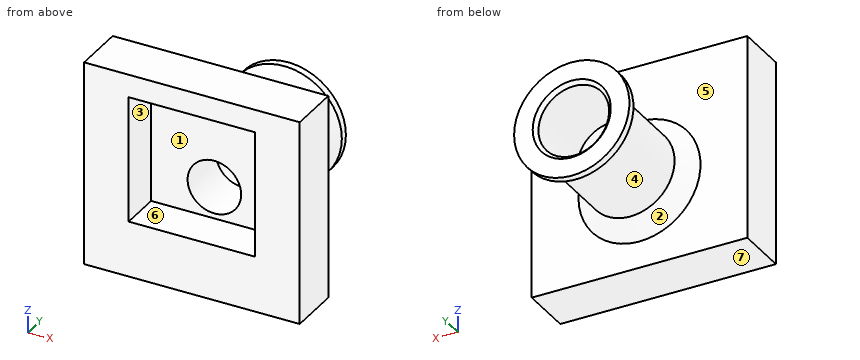
```python
from build123d import *

# Parameters (mm, degrees)
SKETCH2_OUTSIDE_W       = 59.31
SKETCH2_OUTSIDE_H       = 59.31
SKETCH2_OUTSIDE_W_2     = 28.986815524
SKETCH2_OUTSIDE_H_2     = 27.563826398
CUT_EXTRUDE1_DEPTH      = 11
CUT_EXTRUDE1_DEPTH_BACK = 14.593473012
SKETCH3_W               = 17
SKETCH3_H               = 17
CUT_EXTRUDE2_DEPTH      = 6.5


with BuildPart() as part:
    # Sketch1 → Revolve1 (revolve)
    with BuildSketch(Plane.XY):
        Polygon((4.75, 9.5), (4.75, 0), (3.6, -1.15), (3.6, -13.593473012), (22, -13.593473012), (22, -6.593473012), (8.200842899, -6.593473012), (5.95, -4.342630114), (5.95, 7.2), (7.75, 9), (7.75, 10), (5.25, 10), align=None)
    revolve(axis=Axis((0, -12.923275862, 0), (0, 1, 0)))

    # Sketch2 outside → Cut-Extrude1 (cut, two sides)
    with BuildSketch(Plane(origin=(0, 0, 0), x_dir=(1, 0, 0), z_dir=(0, 1, 0))) as cut_extrude1_sk:
        Rectangle(SKETCH2_OUTSIDE_W, SKETCH2_OUTSIDE_H)
        with Locations((0, -2)):
            Rectangle(SKETCH2_OUTSIDE_W_2, SKETCH2_OUTSIDE_H_2, mode=Mode.SUBTRACT)
    extrude(amount=CUT_EXTRUDE1_DEPTH, mode=Mode.SUBTRACT)
    extrude(cut_extrude1_sk.sketch, amount=-CUT_EXTRUDE1_DEPTH_BACK, mode=Mode.SUBTRACT)

    # Sketch3 → Cut-Extrude2 (cut)
    with BuildSketch(Plane(origin=(0, -14.593473012, 0), x_dir=(-1, 0, 0), z_dir=(0, -1, 0))):
        with Locations((0, -4.215)):
            Rectangle(SKETCH3_W, SKETCH3_H)
    extrude(amount=-CUT_EXTRUDE2_DEPTH, mode=Mode.SUBTRACT)


solid = part.part
```
The model under review builds one solid part; all positions refer to its coordinate system, in mm. Face numbers are marked on the shaded views. A direction names the side the tool comes from. Round coordinates to 2 decimals unless told otherwise and drop trailing zeros. Loops run counter-clockwise (first coordinate to the right, second up) from the corner with the lowest first, then second, coordinate; pieces in that order, holes last. Notation, with made-up numbers: (-10.5, -8.75) - (44.5, -8.75) arc R25 ccw to (44.5, 21.25) - close; hole circle Ø1 at (33, 16.5). An arc over 180 degrees is marked (long way). Write each question's results on one line, items separated by ' | '. Start each with the question number.
Q1. Insertion check: P1, Ø7.5, axis at x = 0, z = 0, coming from the -Y side; P2, Ø4, axis at y = 1, z = -5.5, coming from the +X side; P3, Ø12, axis at y = 6, z = 0, coming from the +X side. Each pin has a flat end and moves straight along its axis. Give the tip position at first contact, or say it passes through.
Q2. Take a section at B-B on x = 0. Give the boundary of the cut face in (y, z) (3 decimals), plus the area to 3 significant figures.
Q3. Take a section at D-D on z = -9. Give the boundary of the cut face in (x, y), plus the area to 3 significant figures.
Q4. Tool access review of the marked faces 4, 5, 6 and 7: name each direction out of +Z, -Z, +X, -X, +Y, -Y from which nothing blocks a thin tool from reaching the whole face with its end or side.
Q5. Take a section at A-A on z = 0. Give the boundary of the cut face in (x, y).
Q6. Wall thickness on line 1 along X through (y, z) = (-4.25, 0); line 2 along Z through (x, y) = (0, 3.25): over which ranges is each line inside the solid? List them lowest first. Write a range as [from, to].
Q7. Take a section at C-C on y = 4.5. Give the boundary of the cut face in (x, z).
Q8. Draft analysis for pull direction Y (two halves, no side actions). For the marked faces 1, 2 and 3, state which applies: pulls with the +Y half, pulls with the -Y half, needs draft (parallel to the pull), parting line crosses it, or undercut.
Data:
1) P1: stops at y = -8.09 | P2: stops at x = 4.81 | P3: stops at x = 7.75
2) outline: (-13.593, -11.782) - (-6.593, -11.782) - (-6.593, -8.201) - (-4.343, -5.95) - (7.2, -5.95) - (9, -7.75) - (10, -7.75) - (10, -5.25) - (9.5, -4.75) - (0, -4.75) - (-1.15, -3.6) - (-8.093, -3.6) - (-8.093, -4.285) - (-13.593, -4.285) - close; (-13.593, 12.715) - (-8.093, 12.715) - (-8.093, 3.6) - (-1.15, 3.6) - (0, 4.75) - (9.5, 4.75) - (10, 5.25) - (10, 7.75) - (9, 7.75) - (7.2, 5.95) - (-4.343, 5.95) - (-6.593, 8.201) - (-6.593, 15.782) - (-13.593, 15.782) - close | area: 154 mm²
3) outline: (-14.49, -13.59) - (14.49, -13.59) - (14.49, -6.59) - (-14.49, -6.59) - close | area: 203 mm²
4) face 4: none | face 5: +Y | face 6: -Y | face 7: -Z, +X, -X, +Y, -Y
5) outline: (-14.49, -13.59) - (-8.5, -13.59) - (-8.5, -8.09) - (-3.6, -8.09) - (-3.6, -1.15) - (-4.75, 0) - (-4.75, 9.5) - (-5.25, 10) - (-7.75, 10) - (-7.75, 9) - (-5.95, 7.2) - (-5.95, -4.34) - (-8.2, -6.59) - (-14.49, -6.59) - close; (3.6, -8.09) - (8.5, -8.09) - (8.5, -13.59) - (14.49, -13.59) - (14.49, -6.59) - (8.2, -6.59) - (5.95, -4.34) - (5.95, 7.2) - (7.75, 9) - (7.75, 10) - (5.25, 10) - (4.75, 9.5) - (4.75, 0) - (3.6, -1.15) - close
6) line 1: x = [-5.95, -3.6], [3.6, 5.95] | line 2: z = [-5.95, -4.75], [4.75, 5.95]
7) outline: circle Ø11.9 at (0, 0); hole circle Ø9.5 at (0, 0)
8) face 1: pulls with the -Y half | face 2: undercut | face 3: needs draft
